Could you check a few things on this model? Use its own coordinates, in mm. Give positions to 0.01 mm unless a question says otherwise; leave off trailing zeros. Loops run counter-clockwise (first coordinate to the right, second up) from the corner with the lowest first, then second, coordinate; pieces in that order, holes last. Notation, with made-up numbers: (9, 82.25) - (18, 82.25) arc R12 ccw to (18, 88.25) - close; hole circle Ø11 at (15, 37). An arc over 180 degrees is marked (long way). Write each question's results on one line, items separated by ' | '. Start each with the question number.
1) I want a section at C-C, the plane z = -49.5. Write out the boundary of the cut face in (x, y).
2) I want a section at A-A, the plane x = 3. Write out the boundary of the cut face in (y, z), and give its area (3 significant figures).
3) I want a section at B-B, the plane y = 2.1. Count the separate pieces of the cut face and the enclosed holes in it, and give its area (3 significant figures).
4) If I drill on probe 1 along Z at (x, y) = (29.98, 1.2); probe 2 along Z at (x, y) = (-81, 1.45); probe 3 along Z at (x, y) = (10.5, 1.75), over which ranges is the centre line in solid material (lowest first)? Write a range as [from, to].
5) I'm going to push flat-ended pins straight in: pin 1 (1.5 mm diameter, centred on x = -67, y = 2, fed in from +Z); pin 2 (5 mm diameter, centred on x = 29.98, z = 62.98, fed in from +Y); pin 3 (0.9 mm diameter, centred on x = 75.5, y = 1, fed in from -Z); pin 4 (1.5 mm diameter, centred on y = 1, z = -19, fed in from -X). Where does each tip first touch, or does it pass through?
from build123d import *

# Parameters (mm, degrees)
SKETCH1_W           = 170
SKETCH1_H           = 200
BOSS_EXTRUDE1_DEPTH = 3
SKETCH2_R           = 1.5
CUT_EXTRUDE1_DEPTH  = 43
FILLET1_R           = 30
SKETCH4_W           = 29.4
SKETCH4_H           = 55.8
CUT_EXTRUDE4_DEPTH  = 10
FILLET3_R           = 1
FILLET4_R           = 1
FILLET5_R           = 1
FILLET6_R           = 1
FILLET7_R           = 1
FILLET8_R           = 1
FILLET9_R           = 1
FILLET10_R          = 1
SKETCH5_W           = 25
SKETCH5_H           = 8
CUT_EXTRUDE5_DEPTH  = 10
FILLET11_R          = 2
FILLET12_R          = 2
FILLET13_R          = 2
FILLET14_R          = 2
FILLET15_R          = 2
FILLET16_R          = 2
SKETCH6_R           = 1.5
CUT_EXTRUDE6_DEPTH  = 10
SKETCH7_R           = 1.5
CUT_EXTRUDE8_DEPTH  = 10


with BuildPart() as part:
    # Sketch1 → Boss-Extrude1 (new body)
    with BuildSketch(Plane(origin=(0, 0, 0), x_dir=(1, 0, 0), z_dir=(0, 1, 0))):
        Rectangle(SKETCH1_W, SKETCH1_H)
    extrude(amount=BOSS_EXTRUDE1_DEPTH)

    # Sketch2 → Cut-Extrude1 (cut)
    with BuildSketch(Plane.XZ):
        with Locations((-55, 62.98)):
            Circle(SKETCH2_R)
        with Locations((-55, 29.98)):
            Circle(SKETCH2_R)
        with Locations((-29.98, 62.98)):
            Circle(SKETCH2_R)
        with Locations((-29.98, 29.98)):
            Circle(SKETCH2_R)
        with Locations((29.98, 62.98)):
            Circle(SKETCH2_R)
        with Locations((55, 62.98)):
            Circle(SKETCH2_R)
        with Locations((55, 29.98)):
            Circle(SKETCH2_R)
        with Locations((29.98, 29.98)):
            Circle(SKETCH2_R)
        with Locations((29.98, -62.98)):
            Circle(SKETCH2_R)
        with Locations((29.98, -29.98)):
            Circle(SKETCH2_R)
        with Locations((55, -62.98)):
            Circle(SKETCH2_R)
        with Locations((55, -29.98)):
            Circle(SKETCH2_R)
        with Locations((-29.98, -62.98)):
            Circle(SKETCH2_R)
        with Locations((-55, -62.98)):
            Circle(SKETCH2_R)
        with Locations((-55, -29.98)):
            Circle(SKETCH2_R)
        with Locations((-29.98, -29.98)):
            Circle(SKETCH2_R)
    extrude(amount=-CUT_EXTRUDE1_DEPTH, mode=Mode.SUBTRACT)

    # Fillet1
    fillet1_edges = [part.edges().sort_by_distance(p)[0] for p in [
        (85, 1.5, 100),
        (-85, 1.5, 100),
        (-85, 1.5, -100),
        (85, 1.5, -100),
    ]]
    fillet(fillet1_edges, radius=FILLET1_R)

    # Sketch4 → Cut-Extrude4 (cut)
    with BuildSketch(Plane.XZ):
        with Locations((-82.2, 46.48)):
            Rectangle(SKETCH4_W, SKETCH4_H)
        with Locations((82.2, 46.48)):
            Rectangle(SKETCH4_W, SKETCH4_H)
        with Locations((82.2, -46.48)):
            Rectangle(SKETCH4_W, SKETCH4_H)
        with Locations((-82.2, -46.48)):
            Rectangle(SKETCH4_W, SKETCH4_H)
    extrude(amount=-CUT_EXTRUDE4_DEPTH, mode=Mode.SUBTRACT)

    # Fillet3
    fillet3_edges = [part.edges().sort_by_distance(p)[0] for p in [
        (-84.6785377, 1.5, 74.38),
    ]]
    fillet(fillet3_edges, radius=FILLET3_R)

    # Fillet4
    fillet4_edges = [part.edges().sort_by_distance(p)[0] for p in [
        (-85, 1.5, 18.58),
    ]]
    fillet(fillet4_edges, radius=FILLET4_R)

    # Fillet5
    fillet5_edges = [part.edges().sort_by_distance(p)[0] for p in [
        (84.6785377, 1.5, 74.38),
    ]]
    fillet(fillet5_edges, radius=FILLET5_R)

    # Fillet6
    fillet6_edges = [part.edges().sort_by_distance(p)[0] for p in [
        (85, 1.5, 18.58),
    ]]
    fillet(fillet6_edges, radius=FILLET6_R)

    # Fillet7
    fillet7_edges = [part.edges().sort_by_distance(p)[0] for p in [
        (85, 1.5, -18.58),
    ]]
    fillet(fillet7_edges, radius=FILLET7_R)

    # Fillet8
    fillet8_edges = [part.edges().sort_by_distance(p)[0] for p in [
        (84.6785377, 1.5, -74.38),
    ]]
    fillet(fillet8_edges, radius=FILLET8_R)

    # Fillet9
    fillet9_edges = [part.edges().sort_by_distance(p)[0] for p in [
        (-84.6785377, 1.5, -74.38),
    ]]
    fillet(fillet9_edges, radius=FILLET9_R)

    # Fillet10
    fillet10_edges = [part.edges().sort_by_distance(p)[0] for p in [
        (-85, 1.5, -18.58),
    ]]
    fillet(fillet10_edges, radius=FILLET10_R)

    # Sketch5 → Cut-Extrude5 (cut)
    with BuildSketch(Plane.XZ):
        with Locations((0, -19)):
            Rectangle(SKETCH5_W, SKETCH5_H)
        with Locations((0, 19)):
            Rectangle(SKETCH5_W, SKETCH5_H)
    extrude(amount=-CUT_EXTRUDE5_DEPTH, mode=Mode.SUBTRACT)

    # Fillet11
    fillet11_edges = [part.edges().sort_by_distance(p)[0] for p in [
        (-12.5, 1.5, -23),
        (-12.5, 1.5, -15),
        (12.5, 1.5, -15),
    ]]
    fillet(fillet11_edges, radius=FILLET11_R)

    # Fillet12
    fillet12_edges = [part.edges().sort_by_distance(p)[0] for p in [
        (12.5, 1.5, -23),
    ]]
    fillet(fillet12_edges, radius=FILLET12_R)

    # Fillet13
    fillet13_edges = [part.edges().sort_by_distance(p)[0] for p in [
        (12.5, 1.5, 15),
    ]]
    fillet(fillet13_edges, radius=FILLET13_R)

    # Fillet14
    fillet14_edges = [part.edges().sort_by_distance(p)[0] for p in [
        (12.5, 1.5, 23),
    ]]
    fillet(fillet14_edges, radius=FILLET14_R)

    # Fillet15
    fillet15_edges = [part.edges().sort_by_distance(p)[0] for p in [
        (-12.5, 1.5, 23),
    ]]
    fillet(fillet15_edges, radius=FILLET15_R)

    # Fillet16
    fillet16_edges = [part.edges().sort_by_distance(p)[0] for p in [
        (-12.5, 1.5, 15),
    ]]
    fillet(fillet16_edges, radius=FILLET16_R)

    # Sketch6 → Cut-Extrude6 (cut)
    with BuildSketch(Plane.XZ):
        with Locations((-81, -14.58)):
            Circle(SKETCH6_R)
        with Locations((-81, 14.58)):
            Circle(SKETCH6_R)
        with Locations((-70, 14.58)):
            Circle(SKETCH6_R)
        with Locations((-70, -14.58)):
            Circle(SKETCH6_R)
        with Locations((70, -14.58)):
            Circle(SKETCH6_R)
        with Locations((70, 14.58)):
            Circle(SKETCH6_R)
        with Locations((81, 14.58)):
            Circle(SKETCH6_R)
        with Locations((81, -14.58)):
            Circle(SKETCH6_R)
    extrude(amount=-CUT_EXTRUDE6_DEPTH, mode=Mode.SUBTRACT)

    # Sketch7 → Cut-Extrude8 (cut)
    with BuildSketch(Plane.XZ):
        with Locations((-71.5, 78.38)):
            Circle(SKETCH7_R)
        with Locations((71.5, 78.38)):
            Circle(SKETCH7_R)
        with Locations((71.5, -78.38)):
            Circle(SKETCH7_R)
        with Locations((-71.5, -78.38)):
            Circle(SKETCH7_R)
    extrude(amount=-CUT_EXTRUDE8_DEPTH, mode=Mode.SUBTRACT)


solid = part.part
Answers:
1) outline: (-67.5, 0) - (67.5, 0) - (67.5, 3) - (-67.5, 3) - close
2) outline: (0, -100) - (3, -100) - (3, -23) - (0, -23) - close; (0, -15) - (3, -15) - (3, 15) - (0, 15) - close; (0, 23) - (3, 23) - (3, 100) - (0, 100) - close | area: 552 mm2
3) separate pieces: 1 | enclosed holes: 30 | area: 28,700 mm2
4) probe 1: z = [-100, -64.48], [-61.48, -31.48], [-28.48, 28.48], [31.48, 61.48], [64.48, 100] | probe 2: z = [-84.97, -74.38], [-18.58, -16.08], [-13.08, 13.08], [16.08, 18.58], [74.38, 84.97] | probe 3: z = [-100, -23], [-15, 15], [23, 100]
5) pin 1: stops at z = 97.81 | pin 2: stops at y = 3 | pin 3: stops at z = -92.32 | pin 4: stops at x = -84.74
